For this review, take the finished solid that the model builds, in its own axes (mm). Face numbers are marked on the shaded views. A direction names the side the tool comes from. Coordinates: 2 decimals unless noted, no trailing zeros. Loops run counter-clockwise (first coordinate to the right, second up) from the corner with the lowest first, then second, coordinate; pieces in that order, holes last. Notation, with made-up numbers: (-22, -38) -> (-8, -38) arc R18 ccw to (-8, -31) -> close; hole circle Ø4 at (13, -4). An arc over 180 degrees is marked (long way). Use a Markdown table: item, result.
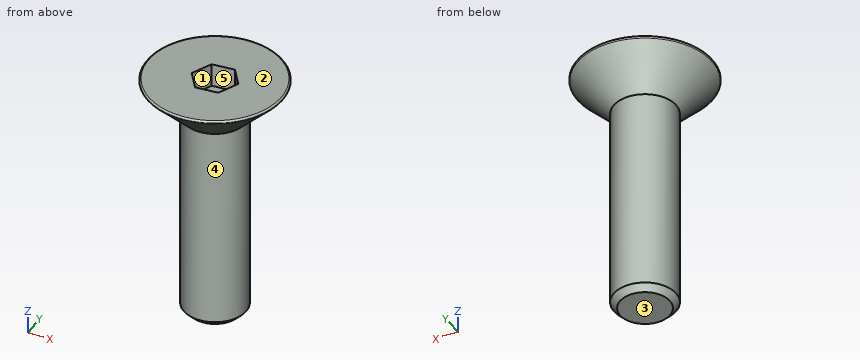
Autodesk Inventor part; units mm, degrees
ref_plane "YZ Plane" through (0, 0, 0) normal (1, 0, 0) x (0, 1, 0)
ref_plane "XZ Plane" through (0, 0, 0) normal (0, 1, 0) x (-1, 0, 0)
ref_plane "XY Plane" through (0, 0, 0) normal (0, 0, 1) x (1, 0, 0)
sketch "Sketch1" plane through (0, 0, 0) normal (0, 0, 1) x (1, 0, 0)
  circle A0 centre (0, 0) radius 2
  dimension "Diameter" = 4
extrude "Extrusion1" add sketch "Sketch1" along normal blind 13.52
sketch "Sketch2" plane through (0, 0, 13.52) normal (0, 0, 1) x (1, 0, 0)
  circle A0 centre (0, 0) radius 2
extrude "Extrusion2" add sketch "Sketch2" along normal blind 2.48 draft 45
sketch "Sketch3" plane through (0, 0, 16) normal (0, 0, 1) x (1, 0, 0)
  circle A0 centre (0, 0) radius 4.48
  circle A1 centre (0, 0) radius 1.4434 construction
  line L0 (0.6042, 1.3108) -> (1.4373, 0.1322)
  line L1 (1.4373, 0.1322) -> (0.8331, -1.1787)
  line L2 (0.8331, -1.1787) -> (-0.6042, -1.3108)
  line L3 (-0.6042, -1.3108) -> (-1.4373, -0.1322)
  line L4 (-1.4373, -0.1322) -> (-0.8331, 1.1787)
  line L5 (-0.8331, 1.1787) -> (0.6042, 1.3108)
  dimension "Hex_Width" = 2.5
extrude "Extrusion3" cut sketch "Sketch3" against normal blind 1.5 contours L0 L1 L2 L3 L4 L5
thread "Thread1"
chamfer "Chamfer2" distance 0.4 angle 45 1 edges at (-2, 0, 0)
fillet "Fillet1" radius 0.1 1 edges at (-4.48, 0, 16)
equation "\"d10\" = Thread_Length"
equation "\"d13\" = Chamfer"
equation "\"Thread_Length\" = 7.52"
properties part number "SCREW, FLAT HD, P, 12.9, M4X0.7X16MM"
(1) For pin 1 Ø5 at (y, z) = (-2.5, 3.5) entering from +X; pin 2 Ø0.8 at (x, y) = (0, 0) entering from +Z; pin 3 Ø1.5 at (x, z) = (-2.5, 5.5) entering from -Y, all flat-tipped, find the tip position at first contact; note any pin that passes through.
Found:
| item | result |
|---|---|
| pin 1 | stops at x = 2 |
| pin 2 | stops at z = 14.5 |
| pin 3 | stops at y = -0.97 |
(2) For line 1 along X through (y, z) = (0, 3.25); line 2 along Y through (x, z) = (-1.5, 10.75); line 3 along Y through (x, z) = (0.25, 1.25), list the stretches that pass through material, from the lowest coordinate up.
Found:
| item | result |
|---|---|
| line 1 | x = -2 to 2 |
| line 2 | y = -1.32 to 1.32 |
| line 3 | y = -1.98 to 1.98 |
(3) Take a section at B-B on z = 5. Write out the cut boundary in (x, y), plus the area to 3 significant figures.
Found:
| item | result |
|---|---|
| outline | circle Ø4 at (0, 0) |
| area | 12.6 mm^2 |
(4) For the marked faces 1 and 2, list the 3-axis set-ups (+Z, -Z, +X, -X, +Y, -Y) from which the entire face can be reached by the end or side of a thin tool; tool diameter is ignored.
Found:
| item | result |
|---|---|
| face 1 | +Z |
| face 2 | +Z, +X, -X, +Y, -Y |
(5) Take a section at A-A on x = 0. Write out the cut boundary in (y, z).
Found:
| item | result |
|---|---|
| outline | (-4.31, 15.83) -> (-2, 13.52) -> (-2, 0.4) -> (-1.6, 0) -> (1.6, 0) -> (2, 0.4) -> (2, 13.52) -> (4.31, 15.83) arc R0.1 ccw to (4.24, 16) -> (1.26, 16) -> (1.26, 14.5) -> (-1.26, 14.5) -> (-1.26, 16) -> (-4.24, 16) arc R0.1 ccw to start |
(6) Mouldability with a two-part tool opening along Y and no side actions: class the marked faces 3, 4 and 5 as pulls with the +Y half, pulls with the -Y half, needs draft (parallel to the pull), parting line crosses it, or undercut.
Found:
| item | result |
|---|---|
| face 3 | needs draft |
| face 4 | parting line crosses it |
| face 5 | undercut |
